Can you work these out from the model? Positions are in its coordinate system, mm. A direction names the side the tool comes from. Coordinates: 2 decimals unless noted, no trailing zeros. Write each loop counter-clockwise with the first axis right and the second up, starting at its lowest first coordinate (ties: lowest second). Pieces come first, ordered by that corner, then holes.
Autodesk Inventor part; units mm, degrees
ref_plane "YZ Plane" through (0, 0, 0) normal (1, 0, 0) x (0, 1, 0)
ref_plane "XZ Plane" through (0, 0, 0) normal (0, 1, 0) x (-1, 0, 0)
ref_plane "XY Plane" through (0, 0, 0) normal (0, 0, 1) x (1, 0, 0)
sketch "Boceto1" plane through (0, 0, 0) normal (0, 1, 0) x (-1, 0, 0)
  line L0 (-100, 40) -> (100, 40)
  line L1 (100, 40) -> (100, -40)
  line L2 (100, -40) -> (-100, -40)
  line L3 (-100, -40) -> (-100, 40)
  line L4 (-100, 40) -> (100, -40) construction
  line L5 (100, 40) -> (-100, -40) construction
  point P0 (0, 0)
  dimension "d0" = 200
  dimension "d1" = 80
extrude "Extrusión1" add sketch "Boceto1" along normal blind 6
sketch "Boceto2" plane through (0, 6, 0) normal (0, 1, 0) x (1, 0, 0)
  line L0 (-67.75, -17.25) -> (87.75, -17.25)
  line L1 (90, -15) -> (90, -15)
  line L2 (87.75, -12.75) -> (-67.75, -12.75)
  line L3 (-70, -15) -> (-70, -15)
  line L4 (0, 0) -> (-99.8063, 0) construction
  line L5 (100, -40) -> (100, 40) construction
  line L6 (100, 40) -> (-100, 40) construction
  line L7 (-100, 40) -> (-100, -40) construction
  line L8 (-100, -40) -> (100, -40) construction
  line L9 (100, -40) -> (100, 40) construction
  arc A0 (-70, -15) -> (-67.75, -17.25) centre (-67.75, -15) ccw
  arc A1 (-67.75, -12.75) -> (-70, -15) centre (-67.75, -15) ccw
  arc A2 (87.75, -17.25) -> (90, -15) centre (87.75, -15) ccw
  arc A3 (90, -15) -> (87.75, -12.75) centre (87.75, -15) ccw
  line L10 (-67.75, 17.25) -> (87.75, 17.25)
  line L11 (87.75, 12.75) -> (-67.75, 12.75)
  arc A4 (-67.75, 17.25) -> (-70, 15) centre (-67.75, 15) ccw
  arc A5 (-70, 15) -> (-67.75, 12.75) centre (-67.75, 15) ccw
  arc A6 (90, 15) -> (87.75, 17.25) centre (87.75, 15) ccw
  arc A7 (87.75, 12.75) -> (90, 15) centre (87.75, 15) ccw
  dimension "d4" = 12.75
  dimension "d5" = 4.5
  dimension "d6" = 10
  dimension "d7" = 30
  dimension "d8" = 2.25
  dimension "d9" = 2.25
  dimension "d10" = 2.25
extrude "Extrusión2" cut sketch "Boceto2" against normal blind 6
sketch "Boceto3" plane through (0, 6, 0) normal (0, 1, 0) x (1, 0, 0)
  line L0 (-67.75, -12.75) -> (87.75, -12.75)
  arc A0 (87.75, -17.25) -> (87.75, -12.75) centre (87.75, -15) ccw
  line L1 (87.75, -17.25) -> (-67.75, -17.25)
  arc A1 (-67.75, -12.75) -> (-67.75, -17.25) centre (-67.75, -15) ccw
  arc A2 (-67.75, 17.25) -> (-67.75, 12.75) centre (-67.75, 15) ccw
  line L2 (-67.75, 17.25) -> (87.75, 17.25)
  arc A3 (87.75, 12.75) -> (87.75, 17.25) centre (87.75, 15) ccw
  line L3 (87.75, 12.75) -> (-67.75, 12.75)
  line L4 (100, 40) -> (-100, 40)
  line L5 (-100, 40) -> (-100, -40)
  line L6 (-100, -40) -> (100, -40)
  line L7 (100, -40) -> (100, 40)
  line L8 (-100, -40) -> (100, -40)
  line L9 (100, -40) -> (100, -50)
  line L10 (100, -50) -> (-100, -50)
  line L11 (-100, -50) -> (-100, -40)
  point P0 (0, 0)
  dimension "d13" = 10
extrude "Extrusión3" add sketch "Boceto3" against normal blind 3 contours L9 L10 L11 L6
sketch "Boceto4" plane through (0, 6, 0) normal (0, 1, 0) x (1, 0, 0)
  line L0 (-100, -50) -> (100, -50)
  line L1 (-100, -45) -> (100, -45) construction
  circle A0 centre (-90, -45) radius 2
  line L2 (-100, 40) -> (-100, -50)
  circle A1 centre (-30, -45) radius 2
  circle A2 centre (30, -45) radius 2
  circle A3 centre (90, -45) radius 2
  point P0 (0, 0)
  dimension "d16" = 5
  dimension "d17" = 4
  dimension "d18" = 10
  dimension "d21" = 60
extrude "Extrusión4" cut sketch "Boceto4" against normal blind 3
properties part number "MesaDePruebas"
1. We'd pull the mould along Z, two halves only. Please class faces 4 (the face through (-1, 3, -40)), 5 (the face through (90, 3, 15)), 6 (the face through (-100, 3, 6)): released by +Z, released by -Z, zero draft, split by the parting line, or undercut.
2. If we section it at A-A, the plane z = -15: List the corners of the cut face in (x, y) for me, plus the area to 3 significant figures.
3. If we section it at B-B, the plane x = 76.5: List the corners of the cut face in (y, z) for me, plus the area to 3 significant figures.
4. Which directions (+Z, -Z, +X, -X, +Y, -Y) give clear straight access to the entire face, cutting with the end or side of a thin tool? Please do faces 1 (the face through (9, 3, 17.25)), 2 (the face through (-1, 6, 4)), 3 (the face through (-1, 3, 45)).
5. If we section it at D-D, the plane x = -73: List the corners of the cut face in (y, z) for me, plus the area to 3 significant figures.
6. If I drill on L1, parallel to Z at x = -45, y = 5.7; L2, parallel to X at y = 4.05, z = 45; L3, parallel to Z at x = 30, y = 4.5, over which ranges is the centre line in solid material (lowest first)?
7. I'm going to push flat-ended pins straight in: P1, Ø3.5, axis at x = -30, z = 45, coming from the +Y side; P2, Ø5, axis at x = 90, z = 45, coming from the +Y side; P3, Ø1.5, axis at x = -12.5, y = 1, coming from the +Z side; P4, Ø3, axis at x = 3, z = 47.5, coming from the -Y side. Where does each tip first touch, or does it pass through?
8. If we section it at C-C, the plane y = 4: List the corners of the cut face in (x, z) for me.
Answers:
1. face 4: released by -Z
1. face 5: undercut
1. face 6: zero draft
2. outline: (-100, 0) - (-70, 0) - (-70, 6) - (-100, 6) - close; (90, 0) - (100, 0) - (100, 6) - (90, 6) - close
2. area: 240 mm2
3. outline: (0, -40) - (6, -40) - (6, -17.25) - (0, -17.25) - close; (0, -12.75) - (6, -12.75) - (6, 12.75) - (0, 12.75) - close; (0, 17.25) - (6, 17.25) - (6, 50) - (3, 50) - (3, 40) - (0, 40) - close
3. area: 456 mm2
4. face 1: +Y, -Y
4. face 2: +Z, -Z, +X, -X, +Y
4. face 3: +Z, +X, -X, -Y
5. outline: (0, -40) - (6, -40) - (6, 50) - (3, 50) - (3, 40) - (0, 40) - close
5. area: 510 mm2
6. L1: z = -40 to -17.25, -12.75 to 12.75, 17.25 to 50
6. L2: x = -100 to -92, -88 to -32, -28 to 28, 32 to 88, 92 to 100
6. L3: z = -40 to -17.25, -12.75 to 12.75, 17.25 to 43, 47 to 50
7. P1: passes through
7. P2: stops at y = 6
7. P3: stops at z = 40
7. P4: stops at y = 3
8. outline: (-100, -40) - (100, -40) - (100, 50) - (-100, 50) - close; hole circle Ø4 at (-90, 45); hole (-67.75, -17.25) - (87.75, -17.25) arc R2.25 ccw to (87.75, -12.75) - (-67.75, -12.75) arc R2.25 ccw to start; hole (-67.75, 12.75) - (87.75, 12.75) arc R2.25 ccw to (87.75, 17.25) - (-67.75, 17.25) arc R2.25 ccw to start; hole circle Ø4 at (-30, 45); hole circle Ø4 at (30, 45); hole circle Ø4 at (90, 45)
